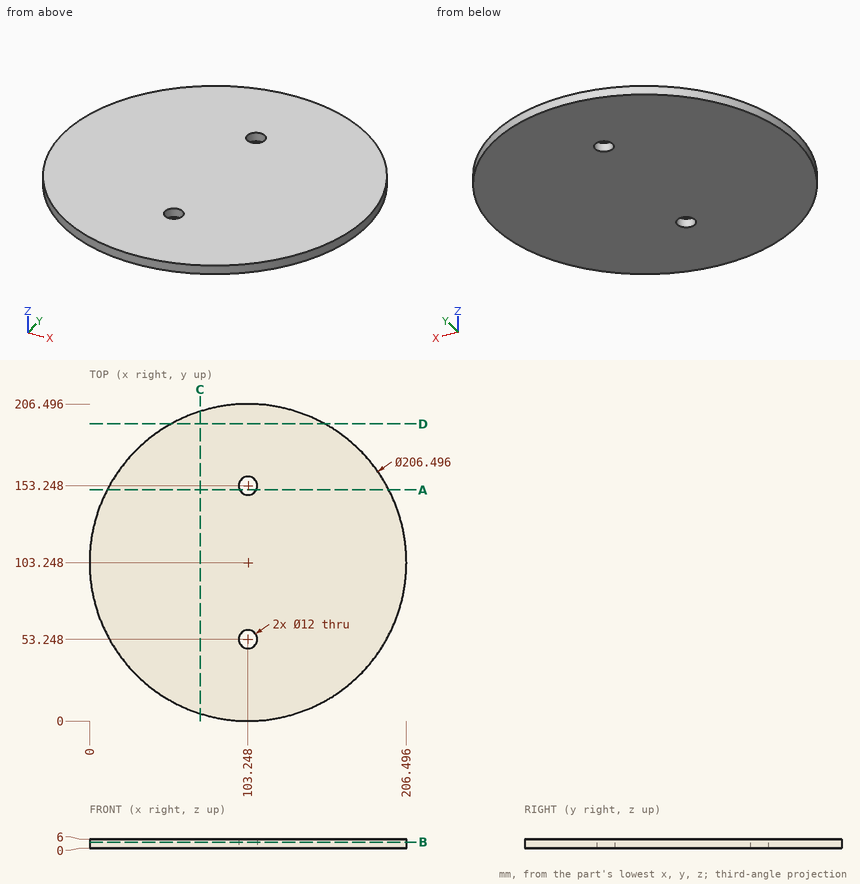
Part print with two shaded views. Sizes in mm from the minimum x, y, z corner. Round coordinates to 2 decimals unless told otherwise and drop trailing zeros. Order: outer loops, then holes, each group sorted by start corner. A loop starts at its lowest first (then second) coordinate and runs counter-clockwise, first axis right, second up. Notation, with made-up numbers: M 46,64.25 L 88,64.25 A24 cw 88,78.25 Z; hole C 69.5,55 d2. An arc over 180 degrees is marked long. Put each result on its own line as item: value. Start each with the question number.
1. Slice it at C-C on x = 72. List the corners of the cut face in (y, z), then the cut area to 3 significant figures.
2. Slice it at A-A on y = 150.5. List the corners of the cut face in (x, z).
3. Slice it at D-D on y = 193.5. List the corners of the cut face in (x, z).
4. Slice it at B-B on z = 4. List the corners of the cut face in (x, y), then the cut area to 3 significant figures.
5. Drill centre lines: probe 1 along X at (y, z) = (55, 2.7); probe 2 along Y at (x, z) = (106.5, 5.55) (1 decimal); probe 3 along Y at (x, z) = (194, 1.3) (1 decimal). Where is each one in solid material? Low to high. Write a range as [from, to].
Findings:
1. outline: M 4.84,0 L 201.65,0 L 201.65,6 L 4.84,6 Z
1. area: 1,180 mm2
2. outline: M 11.45,0 L 97.91,0 L 97.91,6 L 11.45,6 Z; M 108.58,0 L 195.05,0 L 195.05,6 L 108.58,6 Z
3. outline: M 53.1,0 L 153.4,0 L 153.4,6 L 53.1,6 Z
4. outline: C 103.25,103.25 d206.5; hole C 103.25,53.25 d12; hole C 103.25,153.25 d12
4. area: 33,300 mm2
5. probe 1: [11.97, 97.51], [108.99, 194.53]
5. probe 2: [0.1, 48.2], [58.3, 148.2], [158.3, 206.4]
5. probe 3: [54, 152.5]
